Autodesk Inventor part; units mm, degrees
ref_plane "YZ Plane" through (0, 0, 0) normal (1, 0, 0) x (0, 1, 0)
ref_plane "XZ Plane" through (0, 0, 0) normal (0, 1, 0) x (-1, 0, 0)
ref_plane "XY Plane" through (0, 0, 0) normal (0, 0, 1) x (1, 0, 0)
sketch "Sketch1" plane through (0, 0, 0) normal (0, 0, 1) x (1, 0, 0)
  circle A0 centre (0, 0) radius 2.5
  circle A1 centre (0, 0) radius 4.5
  dimension "d0" = 9
  dimension "d1" = 5
extrude "Extrusion1" add sketch "Sketch1" along normal blind 3
sketch "Sketch2" plane through (0, 0, 3) normal (0, 0, 1) x (1, 0, 0)
  circle A0 centre (0, 0) radius 2.5
  circle A1 centre (0, 0) radius 4.5
  circle A2 centre (0, 0) radius 2.95
  circle A3 centre (0, 0) radius 4
  dimension "d4" = 5.9
  dimension "d5" = 0.5
extrude "Extrusion2" cut sketch "Sketch2" against normal blind 0.1 contours A3
sketch "Sketch3" plane through (0, 0, 0) normal (0, 0, -1) x (-1, 0, 0)
  circle A0 centre (0, 0) radius 4
  circle A1 centre (0, 0) radius 2.95
extrude "Extrusion3" cut sketch "Sketch3" against normal blind 0.1
properties part number "9x5x3mm bearing"
Check sheet for the modelled part. Datum: model origin and axes. Units: mm. A direction names the side the tool comes from. Round coordinates to 2 decimals unless told otherwise and drop trailing zeros. Order: outer loops, then holes, each group sorted by start corner. A loop starts at its lowest first (then second) coordinate and runs counter-clockwise, first axis right, second up.
Q1. Draft check along X on faces 4 (the face through (-0.54, 2.44, 1.48)), 5 (the face through (-3, -3, 3)), 6 (the face through (-0.59, -4.46, 1.48)). Enter one of: pulls with the +X half, pulls with the -X half, needs draft (parallel to the pull), parting line crosses it, or undercut.
Filled sheet:
face 4: undercut
face 5: needs draft
face 6: parting line crosses it
Q2. Cross-section at C-C, the plane z = 1.3. Enter the section's corners in (x, y), plus the area to 3 significant figures.
Filled sheet:
outline: circle Ø9 at (0, 0); hole circle Ø5 at (0, 0)
area: 44.0 mm2
Q3. Scan lines: L1, parallel to Y at x = 0, z = 1.55; L2, parallel to Z at x = -3.5, y = 0.5; L3, parallel to X at y = 1.5, z = 0.2. Record each from-to range of solid material in increasing order.
Filled sheet:
L1: y = -4.5 to -2.5, 2.5 to 4.5
L2: z = 0.1 to 2.9
L3: x = -4.24 to -2, 2 to 4.24
Q4. Cross-section at D-D, the plane x = 2.75. Enter the section's corners in (y, z), plus the area to 3 significant figures.
Filled sheet:
outline: (-3.56, 0) - (-2.9, 0) - (-2.9, 0.1) - (-1.07, 0.1) - (-1.07, 0) - (1.07, 0) - (1.07, 0.1) - (2.9, 0.1) - (2.9, 0) - (3.56, 0) - (3.56, 3) - (2.9, 3) - (2.9, 2.9) - (1.07, 2.9) - (1.07, 3) - (-1.07, 3) - (-1.07, 2.9) - (-2.9, 2.9) - (-2.9, 3) - (-3.56, 3) - close
area: 20.6 mm2
Q5. Cross-section at A-A, the plane y = 0. Enter the section's corners in (x, z), plus the area to 3 significant figures.
Filled sheet:
outline: (-4.5, 0) - (-4, 0) - (-4, 0.1) - (-2.95, 0.1) - (-2.95, 0) - (-2.5, 0) - (-2.5, 3) - (-2.95, 3) - (-2.95, 2.9) - (-4, 2.9) - (-4, 3) - (-4.5, 3) - close; (2.5, 0) - (2.95, 0) - (2.95, 0.1) - (4, 0.1) - (4, 0) - (4.5, 0) - (4.5, 3) - (4, 3) - (4, 2.9) - (2.95, 2.9) - (2.95, 3) - (2.5, 3) - close
area: 11.6 mm2
Q6. Depth check by flat-ended pin: P1, Ø5, axis at x = -1, y = 3, coming from the -Z side. Enter the tip coordinate at first touch or a pass-through.
Filled sheet:
P1: stops at z = 0
Q7. Set-up check for faces 1 (the face through (-2, -3, 2.9)), 2 (the face through (2, -3, 0.1)), 3 (the face through (-3, -3, 0)): record each of +Z, -Z, +X, -X, +Y, -Y from which the full face is reachable in a straight line by a thin tool's end or side.
Filled sheet:
face 1: +Z
face 2: -Z
face 3: -Z, +X, -X, +Y, -Y
